Here's how the part is built. I have some questions about the finished solid (model axes, mm). Face numbers are marked on the shaded views. A direction names the side the tool comes from. Round coordinates to 2 decimals unless told otherwise and drop trailing zeros. Loops run counter-clockwise (first coordinate to the right, second up) from the corner with the lowest first, then second, coordinate; pieces in that order, holes last. Notation, with made-up numbers: (49, 64.5) - (77, 64.5) arc R26 ccw to (77, 102.5) - close; hole circle Ø2 at (-19.5, 57). An arc over 180 degrees is marked (long way). Return JSON: item names as keys, results as strings. Group by question number.
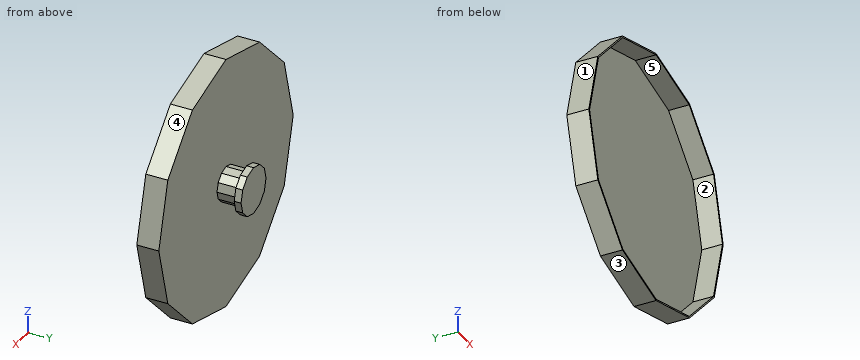
```python
from build123d import *

# Parameters (mm, degrees)
BOSS_EXTRUDE1_DEPTH = 2
BOSS_EXTRUDE2_DEPTH = 30
BOSS_EXTRUDE3_DEPTH = 30
BOSS_EXTRUDE4_DEPTH = 30
BOSS_EXTRUDE5_DEPTH = 10


with BuildPart() as part:
    # Sketch1 → Boss-Extrude1 (new body)
    with BuildSketch(Plane(origin=(0, 0, 0), x_dir=(1, 0, 0), z_dir=(0, 1, 0))):
        Polygon((0, 187.3896103), (-93.69480515, 162.284162925), (-162.284162925, 93.69480515), (-187.3896103, 0), (-162.284162925, -93.69480515), (-93.69480515, -162.284162925), (0, -187.3896103), (93.69480515, -162.284162925), (162.284162925, -93.69480515), (187.3896103, 0), (162.284162925, 93.69480515), (93.69480515, 162.284162925), align=None)
    extrude(amount=BOSS_EXTRUDE1_DEPTH)

    # Sketch2 → Boss-Extrude2 (add)
    with BuildSketch(Plane.XZ):
        Polygon((0, 187.3896103), (-93.69480515, 162.284162925), (-162.284162925, 93.69480515), (-187.3896103, 0), (-162.284162925, -93.69480515), (-93.69480515, -162.284162925), (0, -187.3896103), (93.69480515, -162.284162925), (162.284162925, -93.69480515), (187.3896103, 0), (162.284162925, 93.69480515), (93.69480515, 162.284162925), align=None)
        Polygon((0, 185.319057939), (-92.65952897, 160.491011981), (-160.491011981, 92.65952897), (-185.319057939, 0), (-160.491011981, -92.65952897), (-92.65952897, -160.491011981), (0, -185.319057939), (92.65952897, -160.491011981), (160.491011981, -92.65952897), (185.319057939, 0), (160.491011981, 92.65952897), (92.65952897, 160.491011981), align=None, mode=Mode.SUBTRACT)
    extrude(amount=BOSS_EXTRUDE2_DEPTH)

    # Sketch3 → Boss-Extrude3 (add)
    with BuildSketch(Plane(origin=(0, 2, 0), x_dir=(1, 0, 0), z_dir=(0, 1, 0))):
        Polygon((0, 25.114071484), (-12.557035742, 21.749423897), (-21.749423897, 12.557035742), (-25.114071484, 0), (-21.749423897, -12.557035742), (-12.557035742, -21.749423897), (0, -25.114071484), (12.557035742, -21.749423897), (21.749423897, -12.557035742), (25.114071484, 0), (21.749423897, 12.557035742), (12.557035742, 21.749423897), align=None)
        Polygon((0, 23.043519123), (-11.521759561, 19.956272953), (-19.956272953, 11.521759561), (-23.043519123, 0), (-19.956272953, -11.521759561), (-11.521759561, -19.956272953), (0, -23.043519123), (11.521759561, -19.956272953), (19.956272953, -11.521759561), (23.043519123, 0), (19.956272953, 11.521759561), (11.521759561, 19.956272953), align=None, mode=Mode.SUBTRACT)
    extrude(amount=BOSS_EXTRUDE3_DEPTH)

    # Sketch3<2> → Boss-Extrude4 (add)
    with BuildSketch(Plane(origin=(0, 2, 0), x_dir=(1, 0, 0), z_dir=(0, 1, 0))):
        Polygon((0, 25.114071484), (-12.557035742, 21.749423897), (-21.749423897, 12.557035742), (-25.114071484, 0), (-21.749423897, -12.557035742), (-12.557035742, -21.749423897), (0, -25.114071484), (12.557035742, -21.749423897), (21.749423897, -12.557035742), (25.114071484, 0), (21.749423897, 12.557035742), (12.557035742, 21.749423897), align=None)
        Polygon((0, 23.043519123), (-11.521759561, 19.956272953), (-19.956272953, 11.521759561), (-23.043519123, 0), (-19.956272953, -11.521759561), (-11.521759561, -19.956272953), (0, -23.043519123), (11.521759561, -19.956272953), (19.956272953, -11.521759561), (23.043519123, 0), (19.956272953, 11.521759561), (11.521759561, 19.956272953), align=None, mode=Mode.SUBTRACT)
    extrude(amount=BOSS_EXTRUDE4_DEPTH)

    # Sketch5 → Boss-Extrude5 (add)
    with BuildSketch(Plane(origin=(0, 32, 0), x_dir=(1, 0, 0), z_dir=(0, 1, 0))):
        Polygon((0, 34.773329746), (-17.386664873, 30.114586935), (-30.114586935, 17.386664873), (-34.773329746, 0), (-30.114586935, -17.386664873), (-17.386664873, -30.114586935), (0, -34.773329746), (17.386664873, -30.114586935), (30.114586935, -17.386664873), (34.773329746, 0), (30.114586935, 17.386664873), (17.386664873, 30.114586935), align=None)
    extrude(amount=BOSS_EXTRUDE5_DEPTH)


solid = part.part
```
Q1. If we mould it in two halves opening along Z, with no side actions, what happens to the marked faces 3, 4 and 5? For each: +Z half, -Z half, draft (parallel to the pull), parting line (faces both ways), or undercut.
Q2. Imagine slicing it at A-A, the plane y = -23. List the corners of the cut face in (x, z) for me, and give its area (3 significant figures).
Q3. Will these pins go through, and if not, where does the flat tip stop? pin 1 Ø3 at (x, z) = (89.5, 72.5) entering from +Y; pin 2 Ø10 at (x, y) = (117, -1) entering from -Z; pin 3 Ø1.5 at (x, z) = (-83.5, 96) entering from -Y.
Q4. Imagine slicing it at B-B, the plane x = 4.5. List the corners of the cut face in (y, z) for me.
Q5. Please list where these lines run through material, in increasing order: line 1 (Y direction, x = 167.5, z = 26.5); line 2 (X direction, y = -11.5, z = -57); line 3 (Z direction, x = 58, y = -23).
Q6. Imagine slicing it at C-C, the plane y = 37. List the corners of the cut face in (x, z) for me.
Q7. Imagine slicing it at D-D, the plane x = -130. List the corners of the cut face in (y, z) for me, and give its area (3 significant figures).
Q8. For the marked faces 1 and 2, which set-ups out of +Z, -Z, +X, -X, +Y, -Y let a thin tool reach every point of the face, with its end or its side?
Output values:
{
 "1": {"face 3": "-Z half", "face 4": "+Z half", "face 5": "undercut"},
 "2": {"outline": "(-187.39, 0) - (-162.28, -93.69) - (-93.69, -162.28) - (0, -187.39) - (93.69, -162.28) - (162.28, -93.69) - (187.39, 0) - (162.28, 93.69) - (93.69, 162.28) - (0, 187.39) - (-93.69, 162.28) - (-162.28, 93.69) - close; hole (-185.32, 0) - (-160.49, -92.66) - (-92.66, -160.49) - (0, -185.32) - (92.66, -160.49) - (160.49, -92.66) - (185.32, 0) - (160.49, 92.66) - (92.66, 160.49) - (0, 185.32) - (-92.66, 160.49) - (-160.49, 92.66) - close", "area": "2,320 mm^2"},
 "3": {"pin 1": "stops at y = 2", "pin 2": "stops at z = -143.98", "pin 3": "stops at y = 0"},
 "4": {"outline": "(-30, -186.18) - (2, -186.18) - (2, -23.91) - (32, -23.91) - (32, -33.57) - (42, -33.57) - (42, 33.57) - (32, 33.57) - (32, 23.91) - (2, 23.91) - (2, 186.18) - (-30, 186.18) - (-30, 184.11) - (0, 184.11) - (0, -184.11) - (-30, -184.11) - close; hole (2, -21.84) - (32, -21.84) - (32, 21.84) - (2, 21.84) - close"},
 "5": {"line 1": "y = 0 to 2", "line 2": "x = -172.12 to -170.05, 170.05 to 172.12", "line 3": "z = -171.85 to -169.78, 169.78 to 171.85"},
 "6": {"outline": "(-34.77, 0) - (-30.11, -17.39) - (-17.39, -30.11) - (0, -34.77) - (17.39, -30.11) - (30.11, -17.39) - (34.77, 0) - (30.11, 17.39) - (17.39, 30.11) - (0, 34.77) - (-17.39, 30.11) - (-30.11, 17.39) - close"},
 "7": {"outline": "(-30, -125.98) - (2, -125.98) - (2, 125.98) - (-30, 125.98) - (-30, 123.15) - (0, 123.15) - (0, -123.15) - (-30, -123.15) - close", "area": "674 mm^2"},
 "8": {"face 1": "+Z, -X, +Y, -Y", "face 2": "-Y"}
}
